Check sheet for the modelled part. Datum: model origin and axes. Units: mm. A direction names the side the tool comes from. Give positions to 0.01 mm unless a question says otherwise; leave off trailing zeros. Loops run counter-clockwise (first coordinate to the right, second up) from the corner with the lowest first, then second, coordinate; pieces in that order, holes last. Notation, with made-up numbers: (-8.75, -9) - (35.25, -9) arc R26 cw to (35.25, 19) - close; hole circle Ø8 at (8.5, 5). An arc over 180 degrees is marked (long way). Answer in a Markdown table with one row per item. Add a question column.
(1) Sectioned sample at A-A on z = 8. Enter the section's corners in (x, y).
(2) Sectioned sample at C-C on z = 22. Enter the section's corners in (x, y).
(3) Thickness scan on L1, parallel to Y at x = -2, z = 27; L2, parallel to X at y = 1.15, z = 8; L3, parallel to X at y = -19, z = 15.5. Record the ranges inside material, lowest first.
(4) Draft check along X on faces 4 (the face through (2, -24, 15)), 5 (the face through (-43.373, 1.014, 7.566)), 6 (the face through (-21, 1, 30)). Enter one of: released by +X, released by -X, zero draft, split by the parting line, or undercut.
(5) Sectioned sample at B-B on x = -29.5. Enter the section's corners in (y, z).
(6) Go/stop test with flat-tipped pins: P1, Ø2, axis at x = 0.5, y = -17.5, coming from the -Z side; P2, Ø3.5, axis at x = -41.42, z = 22, coming from the -Y side; P3, Ø0.6, axis at y = -49, z = 19, coming from the -X side; P4, Ø4, axis at y = -14, z = 15.5, coming from the -X side. Record where each tip stops, or that it passes through.
(7) Set-up check for faces 1 (the face through (1, -19, 10)), 2 (the face through (-37, -49, 15)), 3 (the face through (-41, 0, 15)): record each of +Z, -Z, +X, -X, +Y, -Y from which the full face is reachable in a straight line by a thin tool's end or side.
(8) Sectioned sample at D-D on z = 12.5. Enter the section's corners in (x, y), then the cut area to 3 significant figures.
from build123d import *

# Parameters (mm, degrees)
EXTRUDE_1_DEPTH     = 30
SKETCH_3_W          = 10
SKETCH_3_H          = 8
CUT_EXTRUDE_1_DEPTH = 30
SKETCH_4_R          = 2
CUT_EXTRUDE_2_DEPTH = 10


with BuildPart() as part:
    # 草图2 → 拉伸-薄壁1 (new body)
    with BuildSketch(Plane.XY):
        Polygon((-81, 0), (0, 0), (0, -48), (-37, -48), (-37, -50), (2, -50), (2, 2), (-81, 2), align=None)
    extrude(amount=EXTRUDE_1_DEPTH)

    # 草图3 → 切除-拉伸1 (cut)
    with BuildSketch(Plane(origin=(2, 0, 0), x_dir=(0, 0, -1), z_dir=(1, 0, 0))):
        with Locations((-5, -19)):
            Rectangle(SKETCH_3_W, SKETCH_3_H)
    extrude(amount=-CUT_EXTRUDE_1_DEPTH, mode=Mode.SUBTRACT)

    # 草图4 → 切除-拉伸2 (cut)
    with BuildSketch(Plane(origin=(0, 2, 0), x_dir=(1, 0, 0), z_dir=(0, 1, 0))):
        with Locations(Location((-41.420164834, -8, 0), (0, 0, 270))):
            Circle(SKETCH_4_R)
        with Locations(Location((-41.420164834, -22, 0), (0, 0, 270))):
            Circle(SKETCH_4_R)
    extrude(amount=-CUT_EXTRUDE_2_DEPTH, mode=Mode.SUBTRACT)


solid = part.part
Reply:
| question | item | result |
|---|---|---|
| 1 | outline | (-81, 0) - (-43.42, 0) - (-43.42, 2) - (-81, 2) - close; (-39.42, 0) - (0, 0) - (0, -15) - (2, -15) - (2, 2) - (-39.42, 2) - close; (-37, -50) - (2, -50) - (2, -23) - (0, -23) - (0, -48) - (-37, -48) - close |
| 2 | outline | (-81, 0) - (-43.42, 0) - (-43.42, 2) - (-81, 2) - close; (-39.42, 0) - (0, 0) - (0, -48) - (-37, -48) - (-37, -50) - (2, -50) - (2, 2) - (-39.42, 2) - close |
| 3 | L1 | -50 to -48, 0 to 2 |
| 3 | L2 | -81 to -43.42, -39.42 to 2 |
| 3 | L3 | 0 to 2 |
| 4 | face 4 | released by +X |
| 4 | face 5 | undercut |
| 4 | face 6 | zero draft |
| 5 | outline | (-50, 0) - (-48, 0) - (-48, 30) - (-50, 30) - close; (0, 0) - (2, 0) - (2, 30) - (0, 30) - close |
| 6 | P1 | z = 10 |
| 6 | P2 | through |
| 6 | P3 | x = -37 |
| 6 | P4 | x = 0 |
| 7 | face 1 | -Z, +X, -X |
| 7 | face 2 | +Z, -Z, -X, -Y |
| 7 | face 3 | +Z, -Z, -X |
| 8 | outline | (-81, 0) - (0, 0) - (0, -48) - (-37, -48) - (-37, -50) - (2, -50) - (2, 2) - (-81, 2) - close |
| 8 | area | 340 mm^2 |
